Geometry: final body of the model. Coordinates: model frame, mm. A direction names the side the tool comes from. Give positions to 0.01 mm unless a question says otherwise; leave off trailing zeros. Order: outer loops, then holes, each group sorted by start corner. A loop starts at its lowest first (then second) coordinate and runs counter-clockwise, first axis right, second up. Notation, with made-up numbers: (48.25, 52.25) -> (89.25, 52.25) arc R23 cw to (89.25, 80.25) -> close; hole circle Ø11 at (48, 5). An arc over 180 degrees is marked (long way). Answer in a Markdown table with one row per item. Add a question column.
Q1. Contact query for flat-ended pins moving along their axis: P1, Ø5, axis at x = 13.26, z = -13.26, coming from the -Y side; P2, Ø6, axis at x = 4.5, z = 29.5, coming from the +Y side; P3, Ø12, axis at x = 10.5, z = 14.5, coming from the -Y side. Output: stop coordinate, or through.
Q2. Line query: line 1 along Z through (x, y) = (-13, 7.75) (1 decimal); line 2 along X through (y, z) = (3.75, -11.5); line 3 along X through (y, z) = (13.75, 20). Output: solid intervals per line, ascending. Write a range as from..to.
Q3. Set-up query: faces 4 (the face through (14, 8.2, -11.4)), 5 (the face through (15.26, 1.48, 11.28)), 6 (the face through (-16, 13.5, -13)). Return all of +Z, -Z, +X, -X, +Y, -Y with unobstructed straight access to the full face (end or side cutting, diameter ignored); none if empty.
Q4. Pull-direction query (Z, two-part tool) for faces 1 (the face through (0, 18.5, 5)), 2 (the face through (-20, 13.5, 2)), 3 (the face through (-15, 13.5, 15)); classes: +Z half, -Z half, draft (parallel to the pull), parting line (faces both ways), or undercut.
Q5. Cut plane C-C on x = 5.5. Return the cut outline in (y, z).
Q6. Cut plane B-B on y = -1.5. Return the cut outline in (x, z).
Q7. Cut plane A-A on z = -18.75. Return the cut outline in (x, y), and give its area (3 significant figures).
Q8. Cut plane D-D on z = 26. Return the cut outline in (x, y), and give its area (3 significant figures).
from build123d import *
from build123d.topology import SkipClean

# Parameters (mm, degrees)
EXTRUDE_2_DEPTH     = 18.5
EXTRUDE_3_DEPTH     = 37
SKETCH_7_R          = 4
SKETCH_7_R_2        = 2
CUT_EXTRUDE_1_DEPTH = 49.33477026
EXTRUDE_START       = -20.118057
EXTRUDE_5_DEPTH     = 20.118057
SKETCH_9_R          = 25
CUT_EXTRUDE_2_DEPTH = 3
CUT_EXTRUDE_3_REACH = 54.113
SKETCH_10_R         = 20.5
SKETCH_10_R_2       = 18.5
SKETCH_11_R         = 3.5
CUT_EXTRUDE_4_DEPTH = 5
CUT_EXTRUDE_5_DEPTH = 3
SKETCH_13_R         = 10
CUT_EXTRUDE_7_DEPTH = 47.821469602


with BuildPart() as part:
    # 草图1 → 凸台-拉伸2 (new body)
    with BuildSketch(Plane(origin=(0, 0, 0), x_dir=(1, 0, 0), z_dir=(0, 1, 0))):
        with BuildLine():
            ThreePointArc((0, 25), (-17.67766953, 17.67766953), (-25, 0))
            ThreePointArc((-25, 0), (-17.67766953, -17.67766953), (0, -25))
            ThreePointArc((0, -25), (17.67766953, -17.67766953), (25, 0))
            ThreePointArc((25, 0), (17.67766953, 17.67766953), (0, 25))
        make_face()
    extrude(amount=EXTRUDE_2_DEPTH)

    # 草图4 → 凸台-拉伸3 (add)
    with BuildSketch(Plane.XY):
        with BuildLine():
            Line((-18.439088915, 0), (18.439088915, 0))
            ThreePointArc((18.439088915, 0), (0, 17), (-18.439088915, 0))
        make_face()
    extrude(amount=EXTRUDE_3_DEPTH)

    # 草图7 → 切除-拉伸1 (cut, through all)
    with BuildSketch(Plane.XZ):
        with Locations(Location((0, 0, 0), (0, 0, 270))):
            Circle(SKETCH_7_R)
        with Locations(Location((18.75, 0, 0), (0, 0, 270))):
            Circle(SKETCH_7_R_2)
        with Locations(Location((13.258252147, 13.258252147, 0), (0, 0, 270))):
            Circle(SKETCH_7_R_2)
        with Locations(Location((0, 18.75, 0), (0, 0, 90))):
            Circle(SKETCH_7_R_2)
        with Locations(Location((-18.75, 0, 0), (0, 0, 90))):
            Circle(SKETCH_7_R_2)
        with Locations(Location((-13.258252147, 13.258252147, 0), (0, 0, 90))):
            Circle(SKETCH_7_R_2)
        with Locations(Location((13.258252147, -13.258252147, 0), (0, 0, 90))):
            Circle(SKETCH_7_R_2)
        with Locations(Location((0, -18.75, 0), (0, 0, 270))):
            Circle(SKETCH_7_R_2)
        with Locations(Location((-13.258252147, -13.258252147, 0), (0, 0, 270))):
            Circle(SKETCH_7_R_2)
    extrude(amount=-CUT_EXTRUDE_1_DEPTH, mode=Mode.SUBTRACT)

    # 草图8 → 凸台-拉伸5 (add)
    with SkipClean():  # the faces are left unmerged after this step: merging them gives an invalid solid
        with BuildSketch(Plane.XY.offset(37).offset(EXTRUDE_START)):
            with BuildLine():
                Line((-18.439088915, 0), (18.439088915, 0))
                ThreePointArc((18.439088915, 0), (18.5, -1.5), (18.439088915, -3))
                Line((18.439088915, -3), (-18.439088915, -3))
                ThreePointArc((-18.439088915, -3), (-18.5, -1.5), (-18.439088915, 0))
            make_face()
        extrude(amount=EXTRUDE_5_DEPTH)

    # 草图9 → 切除-拉伸2 (cut)
    with SkipClean():  # the faces are left unmerged after this step: merging them gives an invalid solid
        with BuildSketch(Plane.XZ.offset(3)):
            with Locations(Location((0, 0, 0), (0, 0, 137.524279479))):
                Circle(SKETCH_9_R)
        extrude(amount=-CUT_EXTRUDE_2_DEPTH, mode=Mode.SUBTRACT)

    # 切除-拉伸3: up to this face of the body (flat: up to its plane)
    cut_extrude_3_end = Plane(part.part.faces().sort_by_distance((0, 7.168233696, 37))[0])
    # 草图10 → 切除-拉伸3 (cut, up to the picked face)
    with BuildSketch(Plane.XY.offset(16.815171721), mode=Mode.PRIVATE) as cut_extrude_3_sk1:
        with Locations((0, -1.5)):
            Circle(SKETCH_10_R)
        with Locations((0, -1.5)):
            Circle(SKETCH_10_R_2, mode=Mode.SUBTRACT)
    cut_extrude_3_tool1 = split(extrude(cut_extrude_3_sk1.sketch, amount=CUT_EXTRUDE_3_REACH, mode=Mode.PRIVATE), bisect_by=cut_extrude_3_end, keep=Keep.BOTH, mode=Mode.PRIVATE)
    add(cut_extrude_3_tool1.solids().sort_by(Axis((-19.920172, -1.5, 16.815172), (0, 0, 1)))[0], mode=Mode.SUBTRACT)

    # 草图11 → 切除-拉伸4 (cut)
    with SkipClean():  # the faces are left unmerged after this step: merging them gives an invalid solid
        with BuildSketch(Plane(origin=(0, 18.5, 0), x_dir=(1, 0, 0), z_dir=(0, 1, 0))):
            with Locations(Location((0, 18.75, 0), (0, 0, 270))):
                Circle(SKETCH_11_R)
            with Locations(Location((13.258252147, 13.258252147, 0), (0, 0, 270))):
                Circle(SKETCH_11_R)
            with Locations(Location((18.75, 0, 0), (0, 0, 270))):
                Circle(SKETCH_11_R)
            with Locations(Location((13.258252147, -13.258252147, 0), (0, 0, 270))):
                Circle(SKETCH_11_R)
            with Locations(Location((0, -18.75, 0), (0, 0, 270))):
                Circle(SKETCH_11_R)
            with Locations(Location((-13.258252147, -13.258252147, 0), (0, 0, 270))):
                Circle(SKETCH_11_R)
            with Locations(Location((-18.75, 0, 0), (0, 0, 270))):
                Circle(SKETCH_11_R)
            with Locations(Location((-13.258252147, 13.258252147, 0), (0, 0, 270))):
                Circle(SKETCH_11_R)
        extrude(amount=-CUT_EXTRUDE_4_DEPTH, mode=Mode.SUBTRACT)

    # 草图12 → 切除-拉伸5 (cut)
    with SkipClean():  # the faces are left unmerged after this step: merging them gives an invalid solid
        with BuildSketch(Plane.XZ):
            Polygon((0, 22), (-2.814582562, 20.375), (-2.814582562, 17.125), (0, 15.5), (2.814582562, 17.125), (2.814582562, 20.375), align=None)
            Polygon((12.417090251, 16.397511083), (15.556349186, 15.556349186), (16.397511083, 12.417090251), (14.099414044, 10.118993212), (10.960155108, 10.960155108), (10.118993212, 14.099414044), align=None)
            Polygon((-15.556349186, 15.556349186), (-16.397511083, 12.417090251), (-14.099414044, 10.118993212), (-10.960155108, 10.960155108), (-10.118993212, 14.099414044), (-12.417090251, 16.397511083), align=None)
            Polygon((16.397511083, -12.417090251), (15.556349186, -15.556349186), (12.417090251, -16.397511083), (10.118993212, -14.099414044), (10.960155108, -10.960155108), (14.099414044, -10.118993212), align=None)
            Polygon((20.375, 2.814582562), (22, 0), (20.375, -2.814582562), (17.125, -2.814582562), (15.5, 0), (17.125, 2.814582562), align=None)
            Polygon((-17.125, 2.814582562), (-15.5, 0), (-17.125, -2.814582562), (-20.375, -2.814582562), (-22, 0), (-20.375, 2.814582562), align=None)
            Polygon((0, -22), (2.814582562, -20.375), (2.814582562, -17.125), (0, -15.5), (-2.814582562, -17.125), (-2.814582562, -20.375), align=None)
            Polygon((-15.556349186, -15.556349186), (-12.417090251, -16.397511083), (-10.118993212, -14.099414044), (-10.960155108, -10.960155108), (-14.099414044, -10.118993212), (-16.397511083, -12.417090251), align=None)
        extrude(amount=-CUT_EXTRUDE_5_DEPTH, mode=Mode.SUBTRACT)

    # 草图13 → 切除-拉伸7 (cut, through all)
    with SkipClean():  # the faces are left unmerged after this step: merging them gives an invalid solid
        with BuildSketch(Plane.XY.offset(10)):
            Circle(SKETCH_13_R)
        extrude(amount=CUT_EXTRUDE_7_DEPTH, mode=Mode.SUBTRACT)


solid = part.part
Completed:
| question | item | result |
|---|---|---|
| 1 | P1 | stops at y = 3 |
| 1 | P2 | stops at y = 16.94 |
| 1 | P3 | stops at y = 0 |
| 2 | line 1 | z = -21.4..-15.2, -11.3..11.3, 15.2..37 |
| 2 | line 2 | x = -22.2..-14.21, -12.31..12.31, 14.21..22.2 |
| 2 | line 3 | x = -15..-13.7, -10.47..-3.27, 3.27..10.47, 13.7..15 |
| 3 | face 4 | +Y, -Y |
| 3 | face 5 | -Y |
| 3 | face 6 | +Y |
| 4 | face 1 | draft |
| 4 | face 2 | undercut |
| 4 | face 3 | undercut |
| 5 | outline | (0, -24.39) -> (18.5, -24.39) -> (18.5, 24.39) -> (18.25, 24.39) -> (18.25, 16.82) -> (16.16, 16.82) -> (16.16, 37) -> (8.35, 37) -> (8.35, 10) -> (0, 10) -> close |
| 6 | outline | (-18.5, 16.88) -> (-18.44, 16.88) arc R25 cw to (-9.89, 22.96) -> (-9.89, 37) -> (-18.5, 37) -> close; (9.89, 22.96) arc R25 cw to (18.44, 16.88) -> (18.5, 16.88) -> (18.5, 37) -> (9.89, 37) -> close |
| 7 | outline | (-16.54, 0) -> (-2.81, 0) -> (-2.81, 3) -> (-2, 3) -> (-2, 13.5) -> (-3.5, 13.5) -> (-3.5, 18.5) -> (-16.54, 18.5) -> close; (2, 3) -> (2.81, 3) -> (2.81, 0) -> (16.54, 0) -> (16.54, 18.5) -> (3.5, 18.5) -> (3.5, 13.5) -> (2, 13.5) -> close |
| 7 | area | 518 mm² |
| 8 | outline | (-18.44, -3) -> (-9.54, -3) arc R10 cw (long way) to (9.54, -3) -> (18.44, -3) arc R18.5 ccw (long way) to start |
| 8 | area | 377 mm² |
